from build123d import *

# Parameters (mm, degrees)
SKETCH1_R           = 6
BOSS_EXTRUDE1_DEPTH = 5


with BuildPart() as part:
    # Sketch1 → Boss-Extrude1 (new body)
    with BuildSketch(Plane.XY):
        Polygon((-12.885241611, 7.406445139), (-1.954784619, 1.338552), (8.765393483, 7.770658861), (8.555114593, 20.270658861), (-2.3753424, 26.338552), (-13.095520502, 19.906445139), align=None)
        with Locations((-2.165063509, 13.838552)):
            Circle(SKETCH1_R, mode=Mode.SUBTRACT)
    extrude(amount=BOSS_EXTRUDE1_DEPTH)

    # Sketch4 → Cut-Revolve2 (revolve, cut)
    with BuildSketch(Plane(origin=(5.363371252, 9.661359793, 0), x_dir=(0.874312857, -0.48536278, 0), z_dir=(0.48536278, 0.874312857, 0))):
        Polygon((-19.434660926, 0), (-21.111429489, -0.5), (-21.548582722, -0.5), (-21.548582722, 0.495930671), (-19.434660926, 0.495930671), align=None)
    revolve(axis=Axis((-2.164165992, 13.840168751, 0), (0, 0, 1)), mode=Mode.SUBTRACT)


solid = part.part
Read the model definition and answer for the solid it produces. Units are mm, in the model's axes. Coordinates: 2 decimals unless noted, no trailing zeros. Order: outer loops, then holes, each group sorted by start corner. A loop starts at its lowest first (then second) coordinate and runs counter-clockwise, first axis right, second up. Notation, with made-up numbers: M 80.25,85.25 L 93.25,85.25 A35 cw 93.25,122.25 Z; hole C 12,-32.75 d7. An arc over 180 degrees is marked long. Put each result on its own line as item: value. Start each with the question number.
Item 1: Consider probe 1 along Y at (x, z) = (0, 3.55); probe 2 along X at (y, z) = (12.5, 2.35); probe 3 along Y at (x, z) = (-3, 4.1). Determine where each line is inside the solid, lowest interval first. Write a range as [from, to].
Item 2: Given pin 1 Ø9.5 at (x, y) = (-2.17, 13.84) entering from +Z; pin 2 Ø1.5 at (y, z) = (16, 4) entering from -X, each flat-ended and moving along its own axis, determine where each tip first touches the part or whether it passes through.
Item 3: Section A-A, the plane z = 1.25 is taken. Determine the outline of the cut face in (x, y).
Item 4: The mould has two halves that part along X. Classify faces 1 (the face through (3.17, 23.26, 2.47)), 2 (the face through (-5, 20, 5)), 3 (the face through (-3.466, 7.981, 2.465)): +X half, -X half, draft (parallel to the pull), parting line (faces both ways), or undercut.
Computed:
1. probe 1: y = [2.51, 8.24], [19.43, 25.02]
1. probe 2: x = [-12.97, -8.01], [3.68, 8.69]
1. probe 3: y = [1.92, 7.9], [19.78, 25.96]
2. pin 1: passes through
2. pin 2: stops at x = -13.04
3. outline: M -13.1,19.91 L -12.89,7.41 L -1.95,1.34 L 8.77,7.77 L 8.56,20.27 L -2.38,26.34 Z; hole C -2.17,13.84 d12
4. face 1: +X half
4. face 2: draft
4. face 3: undercut
